Check sheet for the modelled part. Datum: model origin and axes. Units: mm. Face numbers are marked on the shaded views. A direction names the side the tool comes from. Round coordinates to 2 decimals unless told otherwise and drop trailing zeros. Loops run counter-clockwise (first coordinate to the right, second up) from the corner with the lowest first, then second, coordinate; pieces in that order, holes last. Notation, with made-up numbers: M -11.75,32 L 3.25,32 A35 ccw 3.25,68 Z; hole C -35,-1 d8. An arc over 180 degrees is marked long. Write item = value, one per line. Start each with the question number.
(1) Scan lines: L1, parallel to X at y = 0, z = 3.55; L2, parallel to X at y = 2, z = 2.05; L3, parallel to X at y = 44.5, z = 4.7. Record each from-to range of solid material in increasing order. Write a range as from..to.
(2) Mould release check, pull along X, two halves, no side actions. Record for the marked faces 3, 4, 5 and 6: pulls with the +X half, pulls with the -X half, needs draft (parallel to the pull), parting line crosses it, or undercut.
(3) Cross-section at C-C on x = 16. Record the boundary of the cut face in (y, z), plus the area to 3 significant figures.
(4) Cross-section at B-B on y = 31. Record the boundary of the cut face in (x, z), plus the area to 3 significant figures.
(5) Cross-section at A-A on z = 3.95. Record the boundary of the cut face in (x, y), plus the area to 3 significant figures.
(6) Set-up check for the marked faces 1 and 2: record each of +Z, -Z, +X, -X, +Y, -Y from which the full face is reachable in a straight line by a thin tool's end or side.
(7) Go/stop test with flat-tipped pins: P1, Ø1, axis at y = 42, z = 4.5, coming from the -X side; P2, Ø2.5, axis at x = 31, y = 1, coming from the -Z side; P3, Ø3, axis at x = 5.5, z = 3, coming from the +Y side. Record where each tip stops, or that it passes through.
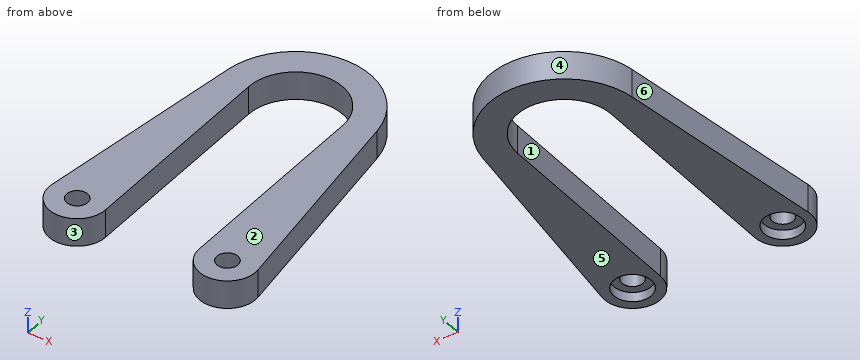
Autodesk Inventor part; units mm, degrees
sketch "スケッチ1" plane through (0, 0, 0) normal (0, 0, 1) x (1, 0, 0)
  line L0 (0, 0) -> (32, 0) construction
  line L1 (0, 60) -> (36, 60) construction
  circle A0 centre (0, 0) radius 2.25
  circle A1 centre (32, 0) radius 2.25
  circle A2 centre (16, 44) radius 10
  circle A3 centre (0, 0) radius 6
  circle A4 centre (32, 0) radius 6
  line L2 (6, 44) -> (6, 0)
  line L3 (26, 44) -> (26, 0)
  line L4 (-5.9466, 0.7988) -> (0.1424, 46.13)
  arc A5 (31.8576, 46.13) -> (0.1424, 46.13) centre (16, 44) ccw
  line L5 (31.8576, 46.13) -> (37.9466, 0.7988)
  point P0 (16, 0)
  dimension "d4" = 4.5
  dimension "d11" = 32
  dimension "d12" = 12
  dimension "d14" = 60
  dimension "d15" = 20
  dimension "d16" = 6
extrude "押し出し1" add sketch "スケッチ1" along normal blind 6 contours A2 L2 A3 L4 A5 L5 A4 L3 | A4 | A3
sketch "スケッチ4" plane through (0, 0, 0) normal (0, 0, -1) x (-1, 0, 0)
  circle A0 centre (-32, 0) radius 2.25 construction
  circle A1 centre (0, 0) radius 2.25 construction
  circle A2 centre (-32, 0) radius 4
  circle A3 centre (0, 0) radius 4
  dimension "d17" = 8
extrude "押し出し3" cut sketch "スケッチ4" against normal blind 2
properties part number "gpu_cable_holder"
Result:
q1.L1 = -6..-2.25, 2.25..6, 26..29.75, 34.25..38
q1.L2 = -5.79..-1.03, 1.03..6, 26..30.97, 33.03..37.79
q1.L3 = -0.08..6.01, 25.99..32.08
q2.face_3 = undercut
q2.face_4 = parting line crosses it
q2.face_5 = needs draft
q2.face_6 = pulls with the -X half
q3.outline = M 54,0 L 60,0 L 60,6 L 54,6 Z
q3.area = 36.0 mm^2
q4.outline = M -1.89,0 L 6,0 L 6,6 L -1.89,6 Z; M 26,0 L 33.89,0 L 33.89,6 L 26,6 Z
q4.area = 94.7 mm^2
q5.outline = M -5.95,0.8 A6 ccw long 6,0 L 6,44 A10 cw 26,44 L 26,0 A6 ccw long 37.95,0.8 L 31.86,46.13 A16 ccw 0.14,46.13 Z; hole C 0,0 d4.5; hole C 32,0 d4.5
q5.area = 1,130 mm^2
q6.face_1 = +Z, -Z, -Y
q6.face_2 = +Z, +X, -X, +Y, -Y
q7.P1 = -0.48
q7.P2 = 2
q7.P3 = 57.23
